Geometry check sheet. Reference: the model listing, model coordinates, mm. Coordinates: 2 decimals unless noted, no trailing zeros. Order: outer loops, then holes, each group sorted by start corner. A loop starts at its lowest first (then second) coordinate and runs counter-clockwise, first axis right, second up. Notation, with made-up numbers: (-9.75, 60) - (36.25, 60) arc R28 cw to (36.25, 94) - close; hole circle Ø2 at (68, 22). An arc over 180 degrees is marked (long way). Return JSON: item names as keys, results as strings. Group by question number.
Item 1: Scan lines: probe 1 along Y at (x, z) = (7, 7.5); probe 2 along Y at (x, z) = (1.25, 5.5); probe 3 along Z at (x, y) = (8.5, 8.75). Record each from-to range of solid material in increasing order.
Item 2: Section check C-C on x = 8. Enter the section's corners in (y, z), then the cut area to 3 significant figures.
Item 3: Section check A-A on z = 7.5. Enter the section's corners in (x, y).
Item 4: Section check B-B on y = 24. Enter the section's corners in (x, z).
Item 5: Draft check along Z on faces 1 (the flat face through (5, 13, 0)), 2 (the flat face through (10, 13, 8)), 3 (the cylindrical face through (5.07, 8.99, 9.34)). Enter one of: pulls with the +Z half, pulls with the -Z half, needs draft (parallel to the pull), parting line crosses it, or undercut.
Autodesk Inventor part; units mm, degrees
ref_plane "YZ Plane" through (0, 0, 0) normal (1, 0, 0) x (0, 1, 0)
ref_plane "XZ Plane" through (0, 0, 0) normal (0, 1, 0) x (-1, 0, 0)
ref_plane "XY Plane" through (0, 0, 0) normal (0, 0, 1) x (1, 0, 0)
sketch "Sketch1" plane through (0, 0, 0) normal (1, 0, 0) x (0, 1, 0)
  line L0 (0, 0) -> (27, 0)
  line L1 (27, 0) -> (27, 15)
  line L2 (27, 15) -> (0, 15)
  line L3 (0, 15) -> (0, 0)
  dimension "d0" = 27
  dimension "d1" = 15
extrude "Extrusion1" add sketch "Sketch1" along normal blind 10
sketch "Sketch2" plane through (10, 0, 0) normal (1, 0, 0) x (0, 0, -1)
  line L0 (0, 27) -> (-15, 27)
  line L1 (-7.5, 27) -> (-7.5, 0)
  line L2 (-15, 0) -> (0, 0)
  line L3 (-10.4795, 25.2) -> (-4.5199, 25.2)
  circle A0 centre (-7.5, 22.6329) radius 2.5
  line L4 (-10.4795, 10) -> (-5, 10)
  circle A1 centre (-7.5, 7.2988) radius 2.5
  dimension "d4" = 1.8
  dimension "d5" = 5
  dimension "d6" = 17
  dimension "d7" = 5
extrude "Extrusion2" cut sketch "Sketch2" against normal blind 10
sketch "Sketch3" plane through (10, 0, 0) normal (1, 0, 0) x (0, 0, -1)
  point P0 (0, 0)
Computed:
{
 "1": {"probe 1": "y = 0 to 4.8, 9.8 to 20.13, 25.13 to 27", "probe 2": "y = 0 to 5.8, 8.8 to 21.13, 24.13 to 27", "probe 3": "z = 0 to 5.46, 9.54 to 15"},
 "2": {"outline": "(0, 0) - (27, 0) - (27, 15) - (0, 15) - close; hole circle Ø5 at (7.3, 7.5); hole circle Ø5 at (22.63, 7.5)", "area": "366 mm²"},
 "3": {"outline": "(0, 0) - (10, 0) - (10, 4.8) - (0, 4.8) - close; (0, 9.8) - (10, 9.8) - (10, 20.13) - (0, 20.13) - close; (0, 25.13) - (10, 25.13) - (10, 27) - (0, 27) - close"},
 "4": {"outline": "(0, 0) - (10, 0) - (10, 5.41) - (0, 5.41) - close; (0, 9.59) - (10, 9.59) - (10, 15) - (0, 15) - close"},
 "5": {"face 1": "pulls with the -Z half", "face 2": "needs draft", "face 3": "undercut"}
}
